Autodesk Inventor part; units mm, degrees
ref_plane "YZ Plane" through (0, 0, 0) normal (1, 0, 0) x (0, 1, 0)
ref_plane "XZ Plane" through (0, 0, 0) normal (0, 1, 0) x (-1, 0, 0)
ref_plane "XY Plane" through (0, 0, 0) normal (0, 0, 1) x (1, 0, 0)
sketch "Sketch2" plane through (0, 0, 0) normal (0, 0, 1) x (1, 0, 0)
  line L0 (-3.5796, 0) -> (-32.4095, 0) construction
  line L1 (-3.5796, 0) -> (-16.3075, 12.7279) construction
  line L2 (-3.5796, 0) -> (-16.3075, -12.7279) construction
  line L3 (-16.3075, 12.7279) -> (-16.3075, -12.7279) construction
  circle A0 centre (-14.5177, 15.8279) radius 1.25
  circle A1 centre (-14.5177, 15.8279) radius 3.1 construction
  circle A2 centre (-19.8871, 12.7279) radius 3.1 construction
  circle A3 centre (-19.8871, 12.7279) radius 1.25
  circle A4 centre (-14.5177, 9.6279) radius 3.1 construction
  circle A5 centre (-14.5177, 9.6279) radius 1.25
  circle A6 centre (-19.4075, -10.9381) radius 1.25
  circle A7 centre (-16.3075, -16.3075) radius 1.25
  circle A8 centre (-13.2075, -10.9381) radius 1.25
  line L4 (-16.3075, 12.7279) -> (-16.3075, -12.7279) construction
  line L5 (-25.3075, 12.7279) -> (-25.3075, -12.7279) construction
  line L6 (-7.3075, -12.7279) -> (-7.3075, 12.7279) construction
  arc A9 (-7.4179, 14.1335) -> (-25.1971, 14.1335) centre (-16.3075, 12.7279) ccw
  arc A10 (-25.1971, -14.1335) -> (-7.4179, -14.1335) centre (-16.3075, -12.7279) ccw
  arc A11 (-7.4179, -14.1335) -> (-7.4179, 14.1335) centre (-96.8075, 0) ccw
  arc A12 (-25.1971, 14.1335) -> (-25.1971, -14.1335) centre (64.1925, 0) ccw
  point P0 (0, 0)
  point P1 (-16.3075, 0)
  point P2 (-16.3075, 0)
  point P3 (-6.3075, 0)
  dimension "d20" = 18
  dimension "d21" = 18
  dimension "d22" = 90
  dimension "d23" = 2.5
  dimension "d24" = 6.2
  dimension "d25" = 360
  dimension "d26" = 2.5
  dimension "d27" = 360
  dimension "d28" = 6.2
  dimension "d29" = 9
  dimension "d31" = 10
extrude "Extrusion1" add sketch "Sketch2" along normal blind 3
chamfer "Chamfer1" distance 1.75 angle 45 3 edges at (-14.4575, -10.9381, 3) (-20.6575, -10.9381, 3) (-17.5575, -16.3075, 3)
sketch "Sketch3" plane through (0, 0, 3) normal (0, 0, 1) x (1, 0, 0)
  circle A0 centre (-14.5177, 9.6279) radius 1.25
  circle A1 centre (-19.8871, 12.7279) radius 1.25
  arc A2 (-7.4179, -14.1335) -> (-7.4179, 14.1335) centre (-96.8075, 0) ccw
  circle A3 centre (-19.4075, -10.9381) radius 3
  circle A4 centre (-13.2075, -10.9381) radius 3
  circle A5 centre (-19.8871, 12.7279) radius 1.25
  circle A6 centre (-14.5177, 15.8279) radius 1.25
  circle A7 centre (-19.4075, -10.9381) radius 3
  circle A8 centre (-14.5177, 15.8279) radius 1.25
  circle A9 centre (-14.5177, 9.6279) radius 1.25
  circle A10 centre (-19.8871, 12.7279) radius 1.25
  arc A11 (-25.1971, -14.1335) -> (-7.4179, -14.1335) centre (-16.3075, -12.7279) ccw
  arc A12 (-7.4179, -14.1335) -> (-7.4179, 14.1335) centre (-96.8075, 0) ccw
  arc A13 (-7.4179, 14.1335) -> (-25.1971, 14.1335) centre (-16.3075, 12.7279) ccw
  arc A14 (-25.1971, 14.1335) -> (-25.1971, -14.1335) centre (64.1925, 0) ccw
  circle A15 centre (-13.2075, -10.9381) radius 3
  circle A16 centre (-16.3075, -16.3075) radius 3
  circle A17 centre (-16.3075, 12.7279) radius 7
  circle A18 centre (-16.3075, -12.7279) radius 8.5
  line L0 (-22.3075, 9.1224) -> (-22.3075, -6.7071)
  line L1 (-10.3075, 9.1224) -> (-10.3075, -6.7071)
  line L2 (-26.3075, 6.5531) -> (-26.3075, -6.806) construction
  line L3 (-6.3075, 6.3529) -> (-6.3075, -7.0063) construction
  point P0 (0, 0)
  dimension "d49" = 17
  dimension "d50" = 14
  dimension "d51" = 4
  dimension "d52" = 4
extrude "Extrusion2" cut sketch "Sketch3" against normal blind 1.5 contours A17 L1 A18 L0
fillet "フィレット1" radius 2 4 edges at (-22.3075, 9.1224, 2.25) (-22.3075, -6.7071, 2.25) (-10.3075, 9.1224, 2.25) (-10.3075, -6.7071, 2.25)
properties part number "クランク_中間" material "Aluminum 2014-T6"
The listing builds one solid part. Answer for the finished solid, in the listing's coordinates (mm). A direction names the side the tool comes from. Give positions to 0.01 mm unless a question says otherwise; leave off trailing zeros. Order: outer loops, then holes, each group sorted by start corner. A loop starts at its lowest first (then second) coordinate and runs counter-clockwise, first axis right, second up. Notation, with made-up numbers: (57, 53) -> (68, 53) arc R27 cw to (68, 85) -> close; hole circle Ø6 at (5.5, 12.25). An arc over 180 degrees is marked (long way). Answer as a JSON object with one key per item and string values. Group by question number.
Item 1: Flat-ended cylindrical pins translate along their axes: pin 1 (4 mm diameter, centred on x = -14.52, y = 9.63, fed in from -Z); pin 2 (3 mm diameter, centred on x = -16.31, y = -16.31, fed in from +Z); pin 3 (1.2 mm diameter, centred on y = -1, z = 2.5, fed in from +X). Find the tip coordinate at first contact, or state that the pin passes through.
Item 2: The part is cut by section B-B on y = -2. Write down the section's boundary in (x, z), and give its area (3 significant figures).
Item 3: Consider L1, parallel to X at y = -10, z = 1.95; L2, parallel to Y at x = -20.5, z = 2.8; L3, parallel to Z at x = -21.75, y = 6. Determine where each line is inside the solid, lowest interval first. Write a range as from..to.
Item 4: Determine the mould class of faces 1 (the flat face through (-16, 0, 0)), 2 (the cylindrical face through (-12.536, -11.992, 0.616)), 3 (the cylindrical face through (-16.129, -21.726, 1.479)) for opening direction Y: pulls with the +Y half, pulls with the -Y half, needs draft (parallel to the pull), parting line crosses it, or undercut.
Item 5: A tool of negligible diameter and unlimited length cuts with its end or side. For faces 4 (the cylindrical face through (-16.486, 21.726, 1.479)), 5 (the flat face through (-10.308, 1, 2)), from which of +Z, -Z, +X, -X, +Y, -Y can it reach the whole face along a straight path? Write none if from no direction.
Item 6: The part is cut by section A-A on z = 2. Write down the section's boundary in (x, y), and give its area (3 significant figures).
Result set:
{
 "1": {"pin 1": "z = 0", "pin 2": "z = 1.5", "pin 3": "x = -6.31"},
 "2": {"outline": "(-26.29, 0) -> (-6.33, 0) -> (-6.33, 3) -> (-10.31, 3) -> (-10.31, 1.5) -> (-22.31, 1.5) -> (-22.31, 3) -> (-26.29, 3) -> close", "area": "41.9 mm²"},
 "3": {"L1": "-25.75..-21.12, -17.7..-14.92, -11.5..-6.86", "L2": "-20.69..-13.52, -8.36..-5.01, 6.66..11.64, 13.82..20.69", "L3": "0..1.5"},
 "4": {"face 1": "needs draft", "face 2": "undercut", "face 3": "pulls with the -Y half"},
 "5": {"face 4": "+Z, -Z, +Y", "face 5": "+Z"},
 "6": {"outline": "(-25.2, -14.13) arc R9 ccw to (-7.42, -14.13) arc R90.5 ccw to (-7.42, 14.13) arc R9 ccw to (-25.2, 14.13) arc R90.5 ccw to start; hole (-22.31, -3.02) arc R2 ccw to (-19.55, -4.87) arc R8.5 cw to (-13.07, -4.87) arc R2 ccw to (-10.31, -3.02) -> (-10.31, 4.67) arc R2 ccw to (-13.2, 6.46) arc R7 cw to (-19.42, 6.46) arc R2 ccw to (-22.31, 4.67) -> close; hole circle Ø4 at (-19.41, -10.94); hole circle Ø2.5 at (-19.89, 12.73); hole circle Ø4 at (-16.31, -16.31); hole circle Ø2.5 at (-14.52, 9.63); hole circle Ø2.5 at (-14.52, 15.83); hole circle Ø4 at (-13.21, -10.94)", "area": "568 mm²"}
}
